Could you check a few things on this drawing? It's one solid part, dimensions in mm from its lowest x, y, z. Give positions to 0.01 mm unless a question says otherwise; leave off trailing zeros. Write each loop counter-clockwise with the first axis right and the second up, starting at its lowest first coordinate (ties: lowest second). Pieces come first, ordered by that corner, then holes. Notation, with made-up numbers: (49, -21) -> (86, -21) arc R19 ccw to (86, 10) -> close; hole circle Ø7 at (14.25, 77). An arc over 180 degrees is marked (long way). Answer as CSV lines item,"result". Start each with the question number.
1. I'm going to push flat-ended pins straight in: P1, Ø1.5, axis at x = 37, z = 78.5, coming from the -Y side; P2, Ø14.5, axis at x = 53.46, y = 42.99, coming from the +Z side. Where does each tip first touch, or does it pass through?
2. I need wall thicknesses on line 1 (Y direction, x = 54, z = 37) (1 decimal); line 2 (Y direction, x = 51, z = 5.5) (1 decimal); line 3 (X direction, y = 42, z = 7.5). Which ranges of each line are inside material? Lowest first, please. Write a range as [from, to].
3. If we section it at A-A on y = 38.5: Write out the boundary of the cut face in (x, z) (1 decimal), plus the area to 3 significant figures.
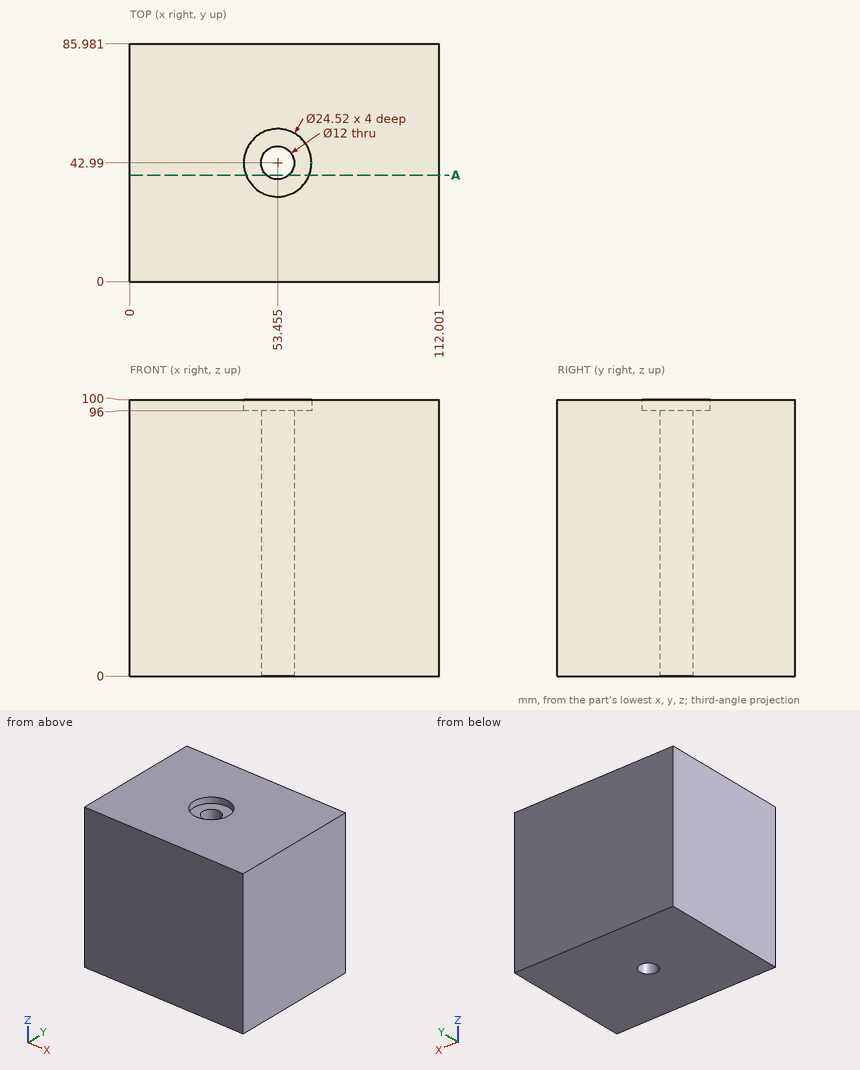
Computed values:
1,P1,"stops at y = 0"
1,P2,"stops at z = 96"
2,line 1,"y = [0, 37], [49, 86]"
2,line 2,"y = [0, 37.5], [48.5, 86]"
2,line 3,"x = [0, 47.54], [59.37, 112]"
3,outline,"(0, 0) -> (49.5, 0) -> (49.5, 96) -> (42, 96) -> (42, 100) -> (0, 100) -> close; (57.4, 0) -> (112, 0) -> (112, 100) -> (64.9, 100) -> (64.9, 96) -> (57.4, 96) -> close"
3,area,"10,300 mm2"
